Can you work these out from the model? Positions are in its coordinate system, mm. Face numbers are marked on the shaded views. A direction names the side the tool comes from. Round coordinates to 2 decimals unless told otherwise and drop trailing zeros. Loops run counter-clockwise (first coordinate to the right, second up) from the corner with the lowest first, then second, coordinate; pieces in that order, holes last.
(1) Thinking about a two-plate mould opening in Z: for the marked faces 4, 5, 6 and 7, which applies, released by +Z, released by -Z, zero draft, split by the parting line, or undercut?
(2) I want a section at A-A on x = -30. Write out the boundary of the cut face in (y, z), plus the area to 3 significant figures.
(3) Which directions (+Z, -Z, +X, -X, +Y, -Y) give clear straight access to the entire face, cutting with the end or side of a thin tool? Please do the marked faces 1, 2 and 3.
(4) If I drill on line 1 along X through (y, z) = (7.5, -20) (3 decimals); line 2 along X through (y, z) = (11.75, -33); line 3 along Y through (x, z) = (-24, -37.15), over which ranges is the centre line in solid material (lowest first)?
(5) I want a section at B-B on z = -29.5. Write out the boundary of the cut face in (x, y).
(6) I want a section at D-D on x = -24. Write out the boundary of the cut face in (y, z).
(7) Will these pins go through, and if not, where does the flat tip stop? pin 1 Ø6.5 at (y, z) = (3.5, -9) entering from -X; pin 2 Ø1.2 at (x, y) = (-24, 6.35) entering from -Z; pin 3 Ø7 at (y, z) = (6, -29) entering from +X.
(8) I want a section at C-C on x = -10. Write out the boundary of the cut face in (y, z).
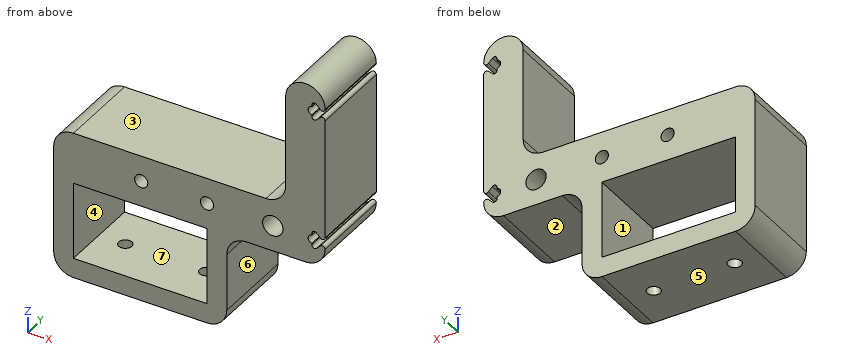
from build123d import *

# Parameters (mm, degrees)
SKETCH1_R           = 1
SKETCH1_R_2         = 1.55
SKETCH1_W           = 20.3
SKETCH1_H           = 11.7
BOSS_EXTRUDE1_DEPTH = 12.7
CUT_EXTRUDE1_REACH  = 63.983
SKETCH2_R           = 1


with BuildPart() as part:
    # Sketch1 → Boss-Extrude1 (new body)
    with BuildSketch(Plane(origin=(0, 0, 0), x_dir=(1, 0, 0), z_dir=(0, 1, 0))):
        with BuildLine():
            Line((-4.055343897, 0.632583633), (-4.075844459, 0.866906139))
            ThreePointArc((-4.075844459, 0.866906139), (-3.83530083, 1.283539926), (-3.361522369, 1.2))
            Line((-3.361522369, 1.2), (-2.761522369, 0.6))
            ThreePointArc((-2.761522369, 0.6), (-2.304491577, 0.509090923), (-2.04560443, 0.89654292))
            Line((-2.04560443, 0.89654292), (-2.04560443, 19.10345708))
            ThreePointArc((-2.04560443, 19.10345708), (-2.304491577, 19.490909077), (-2.761522369, 19.4))
            Line((-2.761522369, 19.4), (-3.361522369, 18.8))
            ThreePointArc((-3.361522369, 18.8), (-3.83530083, 18.716460074), (-4.075844459, 19.133093861))
            Line((-4.075844459, 19.133093861), (-4.055343897, 19.367416367))
            ThreePointArc((-4.055343897, 19.367416367), (-4.635, 20), (-4.055343897, 20.632583633))
            Line((-4.055343897, 20.632583633), (-4.075844459, 20.866906139))
            ThreePointArc((-4.075844459, 20.866906139), (-3.83530083, 21.283539926), (-3.361522369, 21.2))
            Line((-3.361522369, 21.2), (-2.761522369, 20.6))
            ThreePointArc((-2.761522369, 20.6), (-2.304491577, 20.509090923), (-2.04560443, 20.89654292))
            ThreePointArc((-2.04560443, 20.89654292), (-2.924284086, 23.017863263), (-5.04560443, 23.89654292))
            Line((-5.04560443, 23.89654292), (-14, 23.89654292))
            ThreePointArc((-14, 23.89654292), (-16.121320344, 24.775222576), (-17, 26.89654292))
            Line((-17, 26.89654292), (-17, 35.59654292))
            ThreePointArc((-17, 35.59654292), (-17.878679656, 37.717863263), (-20, 38.59654292))
            Line((-20, 38.59654292), (-40.3, 38.59654292))
            ThreePointArc((-40.3, 38.59654292), (-42.421320344, 37.717863263), (-43.3, 35.59654292))
            Line((-43.3, 35.59654292), (-43.3, 19.10345708))
            ThreePointArc((-43.3, 19.10345708), (-42.421320344, 16.982136737), (-40.3, 16.10345708))
            Line((-40.3, 16.10345708), (-11.04560443, 16.10345708))
            ThreePointArc((-11.04560443, 16.10345708), (-8.924284086, 15.224777424), (-8.04560443, 13.10345708))
            Line((-8.04560443, 13.10345708), (-8.04560443, -0.89654292))
            ThreePointArc((-8.04560443, -0.89654292), (-5.04560443, -3.89654292), (-2.04560443, -0.89654292))
            ThreePointArc((-2.04560443, -0.89654292), (-2.304491577, -0.509090923), (-2.761522369, -0.6))
            Line((-2.761522369, -0.6), (-3.361522369, -1.2))
            ThreePointArc((-3.361522369, -1.2), (-3.83530083, -1.283539926), (-4.075844459, -0.866906139))
            Line((-4.075844459, -0.866906139), (-4.055343897, -0.632583633))
            ThreePointArc((-4.055343897, -0.632583633), (-4.635, 0), (-4.055343897, 0.632583633))
        make_face()
        with Locations(Location((-20, 20, 0), (0, 0, 270))):
            Circle(SKETCH1_R, mode=Mode.SUBTRACT)
        with Locations(Location((-10, 20, 0), (0, 0, 270))):
            Circle(SKETCH1_R_2, mode=Mode.SUBTRACT)
        with Locations(Location((-30, 20, 0), (0, 0, 270))):
            Circle(SKETCH1_R, mode=Mode.SUBTRACT)
        with Locations((-30.15, 29.74654292)):
            Rectangle(SKETCH1_W, SKETCH1_H, mode=Mode.SUBTRACT)
    extrude(amount=BOSS_EXTRUDE1_DEPTH)

    # Sketch2 → Cut-Extrude1 (cut, up to next)
    with BuildSketch(Plane(origin=(0, 0, -38.59654292), x_dir=(-1, 0, 0), z_dir=(0, 0, -1)), mode=Mode.PRIVATE) as cut_extrude1_sk1:
        with Locations((36.3, 6.35)):
            Circle(SKETCH2_R)
    cut_extrude1_tool1 = extrude(cut_extrude1_sk1.sketch, amount=-CUT_EXTRUDE1_REACH, mode=Mode.PRIVATE) & part.part
    # Sketch2 → Cut-Extrude1 (cut, up to next)
    with BuildSketch(Plane(origin=(0, 0, -38.59654292), x_dir=(-1, 0, 0), z_dir=(0, 0, -1)), mode=Mode.PRIVATE) as cut_extrude1_sk2:
        with Locations((24, 6.35)):
            Circle(SKETCH2_R)
    cut_extrude1_tool2 = extrude(cut_extrude1_sk2.sketch, amount=-CUT_EXTRUDE1_REACH, mode=Mode.PRIVATE) & part.part
    add(cut_extrude1_tool1.solids().sort_by_distance((-36.3, 6.35, -38.596543))[0], mode=Mode.SUBTRACT)
    add(cut_extrude1_tool2.solids().sort_by_distance((-24, 6.35, -38.596543))[0], mode=Mode.SUBTRACT)


solid = part.part
Filled sheet:
1. face 4: undercut
1. face 5: released by -Z
1. face 6: zero draft
1. face 7: undercut
2. outline: (0, -38.6) - (12.7, -38.6) - (12.7, -35.6) - (0, -35.6) - close; (0, -23.9) - (12.7, -23.9) - (12.7, -21) - (0, -21) - close; (0, -19) - (12.7, -19) - (12.7, -16.1) - (0, -16.1) - close
2. area: 112 mm2
3. face 1: +Y, -Y
3. face 2: -Z, +X, +Y, -Y
3. face 3: +Z, -X, +Y, -Y
4. line 1: x = -43.3 to -31, -29 to -21, -19 to -11.55, -8.45 to -4.635
4. line 2: x = -43.3 to -40.3, -20 to -17
4. line 3: y = 0 to 5.35, 7.35 to 12.7
5. outline: (-43.3, 0) - (-40.3, 0) - (-40.3, 12.7) - (-43.3, 12.7) - close; (-20, 0) - (-17, 0) - (-17, 12.7) - (-20, 12.7) - close
6. outline: (0, -38.6) - (5.35, -38.6) - (5.35, -35.6) - (0, -35.6) - close; (0, -23.9) - (12.7, -23.9) - (12.7, -16.1) - (0, -16.1) - close; (7.35, -38.6) - (12.7, -38.6) - (12.7, -35.6) - (7.35, -35.6) - close
7. pin 1: stops at x = -8.05
7. pin 2: stops at z = -23.9
7. pin 3: stops at x = -16.66
8. outline: (0, -23.9) - (12.7, -23.9) - (12.7, -21.55) - (0, -21.55) - close; (0, -18.45) - (12.7, -18.45) - (12.7, -15.92) - (0, -15.92) - close
